```python
from build123d import *

# Parameters (mm, degrees)
SKETCH1_W                 = 35.000000224
SKETCH1_H                 = 10
BOSS_EXTRUDE1_DEPTH       = 5
CUT_EXTRUDE1_DEPTH        = 15.000000224
SKETCH3_W                 = 20
SKETCH3_H                 = 5
BOSS_EXTRUDE2_DEPTH       = 5
CUT_EXTRUDE2_DEPTH        = 15.000000224
SKETCH5_W                 = 20
SKETCH5_H                 = 5
BOSS_EXTRUDE3_DEPTH       = 5
BOSS_EXTRUDE4_DEPTH       = 15
BOSS_EXTRUDE5_DEPTH       = 15
BOSS_EXTRUDE6_DEPTH       = 15
CUT_EXTRUDE3_DEPTH        = 1
SKETCH10_W                = 15
SKETCH10_H                = 1.5
CUT_EXTRUDE4_DEPTH        = 2.000000104
SKETCH11_W                = 2.000000194
SKETCH11_H                = 1.5
CUT_EXTRUDE5_DEPTH        = 15
SKETCH12_W                = 1.5
SKETCH12_H                = 2
CUT_EXTRUDE6_DEPTH        = 15.000000224
SKETCH13_W                = 1.5
SKETCH13_H                = 2.000000104
CUT_EXTRUDE7_DEPTH        = 15.000000224
SKETCH14_W                = 1.999999806
SKETCH14_H                = 1.5
CUT_EXTRUDE8_DEPTH        = 15
SKETCH15_W                = 1.5
SKETCH15_H                = 15
CUT_EXTRUDE9_DEPTH        = 2.000000104
SKETCH16_W                = 1.5
SKETCH16_H                = 15
CUT_EXTRUDE10_DEPTH       = 2
SKETCH17_W                = 1.999999806
SKETCH17_H                = 1.5
CUT_EXTRUDE11_DEPTH       = 15
F_6_CLEARANCE_HOLE1_D     = 4
F_6_CLEARANCE_HOLE1_DEPTH = 5
F_6_CLEARANCE_HOLE2_D     = 4
F_6_CLEARANCE_HOLE2_DEPTH = 35
F_6_CLEARANCE_HOLE3_D     = 4
F_6_CLEARANCE_HOLE3_DEPTH = 35.000000224
FILLET1_R                 = 2


with BuildPart() as part:
    # Sketch1 → Boss-Extrude1 (new body)
    with BuildSketch(Plane(origin=(0, 0, -5), x_dir=(-1, 0, 0), z_dir=(0, 0, -1))):
        with Locations((-2.499999888, 10)):
            Rectangle(SKETCH1_W, SKETCH1_H)
    extrude(amount=-BOSS_EXTRUDE1_DEPTH)

    # Sketch2 → Cut-Extrude1 (cut)
    with BuildSketch(Plane.ZY.offset(15.000000224)):
        Polygon((-3, 5), (-5, 7), (-5, 5), align=None)
    extrude(amount=-CUT_EXTRUDE1_DEPTH, mode=Mode.SUBTRACT)

    # Sketch3 → Boss-Extrude2 (add)
    with BuildSketch(Plane.XZ.offset(-5)):
        with Locations((10, -2.5)):
            Rectangle(SKETCH3_W, SKETCH3_H)
    extrude(amount=BOSS_EXTRUDE2_DEPTH)

    # Sketch4 → Cut-Extrude2 (cut)
    with BuildSketch(Plane.ZY.offset(15.000000224)):
        Polygon((-5, 13), (-3, 15), (-5, 15), align=None)
    extrude(amount=-CUT_EXTRUDE2_DEPTH, mode=Mode.SUBTRACT)

    # Sketch5 → Boss-Extrude3 (add)
    with BuildSketch(Plane(origin=(0, 15, 0), x_dir=(-1, 0, 0), z_dir=(0, 1, 0))):
        with Locations((-10, -2.5)):
            Rectangle(SKETCH5_W, SKETCH5_H)
    extrude(amount=BOSS_EXTRUDE3_DEPTH)

    # Sketch6 → Boss-Extrude4 (add)
    with BuildSketch(Plane.XZ):
        Polygon((15, 0), (15, -3), (13, -5), (7, -5), (5, -3), (5, 0), align=None)
    extrude(amount=BOSS_EXTRUDE4_DEPTH)

    # Sketch7 → Boss-Extrude5 (add)
    with BuildSketch(Plane(origin=(0, 0, -5), x_dir=(-1, 0, 0), z_dir=(0, 0, -1))):
        Polygon((-5, 20), (-5, 17), (-7, 15), (-13, 15), (-15, 17), (-15, 20), align=None)
    extrude(amount=BOSS_EXTRUDE5_DEPTH)

    # Sketch8 → Boss-Extrude6 (add)
    with BuildSketch(Plane(origin=(0, 0, -5), x_dir=(-1, 0, 0), z_dir=(0, 0, -1))):
        Polygon((-20, 5), (-20, 15), (-17, 15), (-15, 13), (-15, 7), (-17, 5), align=None)
    extrude(amount=BOSS_EXTRUDE6_DEPTH)

    # Sketch9 → Cut-Extrude3 (cut)
    with BuildSketch(Plane(origin=(0, 0, -5), x_dir=(-1, 0, 0), z_dir=(0, 0, -1))):
        Polygon((-16.000000238, 16), (-16.000000238, 14.000000238), (-15, 13), (-15, 7), (-16.000000238, 5.999999762), (-16.000000238, 4), (-4, 4), (-4, 16), (-6, 16), (-7, 15), (-13, 15), (-14, 16), align=None)
    extrude(amount=-CUT_EXTRUDE3_DEPTH, mode=Mode.SUBTRACT)

    # Sketch10 → Cut-Extrude4 (cut)
    with BuildSketch(Plane.ZY.offset(-5)):
        with Locations((-12.5, 19.25)):
            Rectangle(SKETCH10_W, SKETCH10_H)
    extrude(amount=-CUT_EXTRUDE4_DEPTH, mode=Mode.SUBTRACT)

    # Sketch11 → Cut-Extrude5 (cut)
    with BuildSketch(Plane.XZ.offset(15)):
        with Locations((6.000000097, -0.75)):
            Rectangle(SKETCH11_W, SKETCH11_H)
    extrude(amount=-CUT_EXTRUDE5_DEPTH, mode=Mode.SUBTRACT)

    # Sketch12 → Cut-Extrude6 (cut)
    with BuildSketch(Plane.ZY.offset(15.000000224)):
        with Locations((-0.75, 14)):
            Rectangle(SKETCH12_W, SKETCH12_H)
    extrude(amount=-CUT_EXTRUDE6_DEPTH, mode=Mode.SUBTRACT)

    # Sketch13 → Cut-Extrude7 (cut)
    with BuildSketch(Plane.ZY.offset(15.000000224)):
        with Locations((-0.75, 6.000000052)):
            Rectangle(SKETCH13_W, SKETCH13_H)
    extrude(amount=-CUT_EXTRUDE7_DEPTH, mode=Mode.SUBTRACT)

    # Sketch14 → Cut-Extrude8 (cut)
    with BuildSketch(Plane.XZ.offset(15)):
        with Locations((14.000000097, -0.75)):
            Rectangle(SKETCH14_W, SKETCH14_H)
    extrude(amount=-CUT_EXTRUDE8_DEPTH, mode=Mode.SUBTRACT)

    # Sketch15 → Cut-Extrude9 (cut)
    with BuildSketch(Plane.XZ.offset(-5)):
        with Locations((19.25, -12.5)):
            Rectangle(SKETCH15_W, SKETCH15_H)
    extrude(amount=-CUT_EXTRUDE9_DEPTH, mode=Mode.SUBTRACT)

    # Sketch16 → Cut-Extrude10 (cut)
    with BuildSketch(Plane(origin=(0, 15, 0), x_dir=(-1, 0, 0), z_dir=(0, 1, 0))):
        with Locations((-19.25, -12.5)):
            Rectangle(SKETCH16_W, SKETCH16_H)
    extrude(amount=-CUT_EXTRUDE10_DEPTH, mode=Mode.SUBTRACT)

    # Sketch17 → Cut-Extrude11 (cut)
    with BuildSketch(Plane(origin=(0, 0, -20), x_dir=(-1, 0, 0), z_dir=(0, 0, -1))):
        with Locations((-14.000000097, 19.25)):
            Rectangle(SKETCH17_W, SKETCH17_H)
    extrude(amount=-CUT_EXTRUDE11_DEPTH, mode=Mode.SUBTRACT)

    # #6 Clearance Hole1
    with Locations(Plane(origin=(0, 0, -5), x_dir=(-1, 0, 0), z_dir=(0, 0, -1))):
        with Locations((-10, -9.5), (9.5, 10)):
            Hole(F_6_CLEARANCE_HOLE1_D / 2, depth=F_6_CLEARANCE_HOLE1_DEPTH)

    # #6 Clearance Hole2
    with Locations(Plane(origin=(0, 20, 0), x_dir=(1, 0, 0), z_dir=(0, 1, 0))):
        with Locations((10.000000149, 14.5)):
            Hole(F_6_CLEARANCE_HOLE2_D / 2, depth=F_6_CLEARANCE_HOLE2_DEPTH)

    # #6 Clearance Hole3
    with Locations(Plane(origin=(20, 0, 0), x_dir=(0, 0, -1), z_dir=(1, 0, 0))):
        with Locations((14.5, 10.000000052)):
            Hole(F_6_CLEARANCE_HOLE3_D / 2, depth=F_6_CLEARANCE_HOLE3_DEPTH)

    # Fillet1
    fillet1_edges = [part.edges().sort_by_distance(p)[0] for p in [
        (20, 0, -2.5),
        (0, 0, -2.5),
        (0, 20, -2.5),
        (20, 20, -2.5),
    ]]
    fillet(fillet1_edges, radius=FILLET1_R)


solid = part.part
```
Geometry: final body of the model. Coordinates: model frame, mm. A direction names the side the tool comes from. Coordinates: 2 decimals unless noted, no trailing zeros. Loops run counter-clockwise (first coordinate to the right, second up) from the corner with the lowest first, then second, coordinate; pieces in that order, holes last. Notation, with made-up numbers: (29, -9.5) -> (59, -9.5) arc R27 ccw to (59, 14.5) -> close; hole circle Ø1 at (78, 0). An arc over 180 degrees is marked (long way). Use a Markdown table: item, result. Add a question column.
(1) Line query: line 1 along X through (y, z) = (17.25, -14.5); line 2 along X through (y, z) = (10, -19); line 3 along Y through (x, z) = (-5, -1). Output: solid intervals per line, ascending.
(2) Section query B-B, the plane z = -9.5. Return loops of the section in (x, y), plus the area to 3 significant figures.
(3) Access query for faces 1 (the flat face through (6, -7, -4)), 2 (the flat face through (15, 10, -12)), 3 (the flat face through (-7, 15, -2)), 4 (the flat face through (5, -7, -2)). Directions: +Z, -Z, +X, -X, +Y, -Y. A direction counts if a zero-diameter tool reaches every point of the face in a straight line with its end or side. Return the directions, or none.
(4) Pin query (flat end, axial travel): pin 1 Ø0.5 at (x, z) = (4.5, -4.5) entering from -Y; pin 2 Ø1.2 at (x, z) = (17.5, -11) entering from +Y; pin 3 Ø0.5 at (y, z) = (15.5, -4.5) entering from -X; pin 4 Ø2.5 at (x, z) = (10, -14.5) entering from +Y. Return the tip coordinate at first contact, or that it passes through.
(5) Section query A-A, the plane y = 10. Return loops of the section in (x, z), plus the area to 3 significant figures.
(6) Mould query, pull axis Y, two halves, no side actions, for faces 5 (the flat face through (16, 5, -4.5)), 6 (the flat face through (10, 10, -4)), 7 (the cylindrical face through (19.43, 19.4, -2.46)), 8 (the flat face through (13, -8, -1)). Classes: pulls with the +Y half, pulls with the -Y half, needs draft (parallel to the pull), parting line crosses it, or undercut.
(7) Section query C-C, the plane x = -9.5. Return loops of the section in (y, z), plus the area to 3 significant figures.
Answer:
| question | item | result |
|---|---|---|
| 1 | line 1 | x = 5 to 8, 12 to 15 |
| 1 | line 2 | x = 15 to 20 |
| 1 | line 3 | y = 7 to 13 |
| 2 | outline | (5, 17) -> (7, 15) -> (13, 15) -> (15, 17) -> (15, 18.5) -> (13, 18.5) -> (13, 20) -> (7, 20) -> (7, 18.5) -> (5, 18.5) -> close; (15, 7) -> (17, 5) -> (18.5, 5) -> (18.5, 7) -> (20, 7) -> (20, 13) -> (18.5, 13) -> (18.5, 15) -> (17, 15) -> (15, 13) -> close |
| 2 | area | 80.0 mm^2 |
| 3 | face 1 | -Z, -X, -Y |
| 3 | face 2 | -Z |
| 3 | face 3 | +Z, -Z, -X, +Y |
| 3 | face 4 | +Z, -Z, -X, -Y |
| 4 | pin 1 | stops at y = 0 |
| 4 | pin 2 | stops at y = 15 |
| 4 | pin 3 | stops at x = 0 |
| 4 | pin 4 | passes through |
| 5 | outline | (-15, -5) -> (-11.5, -5) -> (-11.5, 0) -> (-15, 0) -> close; (-7.5, -5) -> (4, -5) -> (4, -4) -> (15, -4) -> (15, -12.5) -> (20, -12.5) -> (20, 0) -> (-7.5, 0) -> close; (15, -20) -> (20, -20) -> (20, -16.5) -> (15, -16.5) -> close |
| 5 | area | 199 mm^2 |
| 6 | face 5 | undercut |
| 6 | face 6 | undercut |
| 6 | face 7 | pulls with the +Y half |
| 6 | face 8 | needs draft |
| 7 | outline | (5, -3) -> (7, -5) -> (8, -5) -> (8, 0) -> (7, 0) -> (7, -1.5) -> (5, -1.5) -> close; (12, -5) -> (13, -5) -> (15, -3) -> (15, -1.5) -> (13, -1.5) -> (13, 0) -> (12, 0) -> close |
| 7 | area | 20.0 mm^2 |
